Design review of the part built by this model. Coordinates are the model's own, in mm. Face numbers are marked on the shaded views. A direction names the side the tool comes from. Coordinates: 2 decimals unless noted, no trailing zeros. Write each loop counter-clockwise with the first axis right and the second up, starting at its lowest first coordinate (ties: lowest second). Pieces come first, ordered by that corner, then holes. Notation, with made-up numbers: (89, 24.5) - (134, 24.5) arc R25 cw to (134, 48.5) - close; hole circle Ø4 at (-38, 39.5). An arc over 180 degrees is marked (long way). Answer as a JSON object with one key per item and string values.
```python
from build123d import *

# Parameters (mm, degrees)
EXTRUDE_2_DEPTH     = 30
SKETCH_5_R          = 1.498354352
EXTRUDE_3_DEPTH     = 5
SKETCH_6_R          = 1.5
CUT_EXTRUDE_1_DEPTH = 5


with BuildPart() as part:
    # 草图4 → 凸台-拉伸2 (new body)
    with BuildSketch(Plane.XY):
        Polygon((1.108848503, -2.025780919), (2.30880199, -0.052599487), (1.199953487, 1.973181432), (-1.108848503, 2.025780919), (-2.30880199, 0.052599487), (-1.199953487, -1.973181432), align=None)
    extrude(amount=EXTRUDE_2_DEPTH)

    # 草图5 → 凸台-拉伸3 (add)
    with BuildSketch(Plane(origin=(0, 0, 0), x_dir=(-1, 0, 0), z_dir=(0, 0, -1))):
        Circle(SKETCH_5_R)
    extrude(amount=EXTRUDE_3_DEPTH)

    # 草图6 → 切除-拉伸1 (cut)
    with BuildSketch(Plane.XY.offset(30)):
        Circle(SKETCH_6_R)
    extrude(amount=-CUT_EXTRUDE_1_DEPTH, mode=Mode.SUBTRACT)


solid = part.part
```
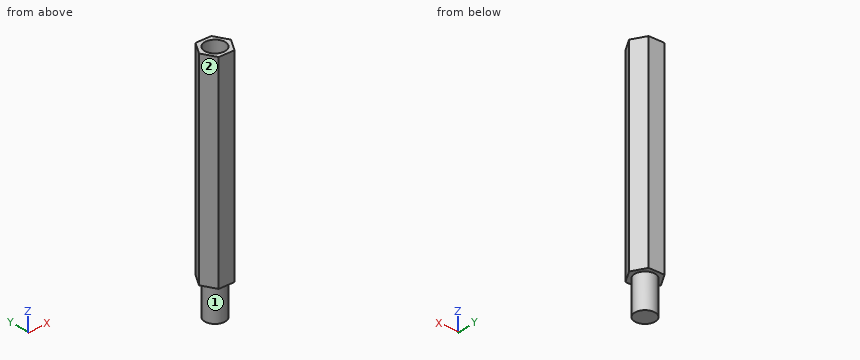
(1) To check wall thickness, follow line 1 (Z direction, x = 1.1, y = 1.55); line 2 (Z direction, x = -1.05, y = 0.3); line 3 (Y direction, x = 0, z = 26.25). State the ranges of each line that lie inside material, in increasing order. Write a range as from..to.
Solved:
{"line 1": "z = 0..30", "line 2": "z = -5..25", "line 3": "y = -2..-1.5, 1.5..2"}
(2) Tool access review of the marked faces 1 and 2: name each direction out of +Z, -Z, +X, -X, +Y, -Y from which nothing blocks a thin tool from reaching the whole face with its end or side.
Solved:
{"face 1": "-Z", "face 2": "+Z, -Z, -X, -Y"}
(3) Take a section at B-B, the plane x = -0.6. Write out the cut boundary in (y, z), and give its area (3 significant figures).
Solved:
{"outline": "(-1.99, 0) - (-1.37, 0) - (-1.37, -5) - (1.37, -5) - (1.37, 0) - (2.01, 0) - (2.01, 30) - (1.37, 30) - (1.37, 25) - (-1.37, 25) - (-1.37, 30) - (-1.99, 30) - close", "area": "120 mm^2"}
(4) Take a section at C-C, the plane z = 16.5. Write out the cut boundary in (x, y).
Solved:
{"outline": "(-2.31, 0.05) - (-1.2, -1.97) - (1.11, -2.03) - (2.31, -0.05) - (1.2, 1.97) - (-1.11, 2.03) - close"}
(5) Take a section at A-A, the plane z = 25.5. Write out the cut boundary in (x, y).
Solved:
{"outline": "(-2.31, 0.05) - (-1.2, -1.97) - (1.11, -2.03) - (2.31, -0.05) - (1.2, 1.97) - (-1.11, 2.03) - close; hole circle Ø3 at (0, 0)"}
